The drawing under review shows one solid part. Ordinate dimensions are in mm from its lowest x, y, z. A direction names the side the tool comes from. Round coordinates to 2 decimals unless told otherwise and drop trailing zeros. Write each loop counter-clockwise with the first axis right and the second up, starting at its lowest first coordinate (ties: lowest second). Pieces come first, ordered by that corner, then holes. Notation, with made-up numbers: (62, 20) -> (69, 20) arc R24 cw to (69, 51) -> close; hole circle Ø5 at (21.25, 19.5). An arc over 180 degrees is marked (long way). Use CSV: the item, a comma, the result in double quotes. Start each with the question number.
1) Machinability: for the marked faces 1, 2, 3, 4 and 5, which of the approach directions +Z, -Z, +X, -X, +Y, -Y give a long, thin tool a straight path to every point of the face, cutting with its end or side? Answer none if there is none.
2) Take a section at B-B, the plane y = 62.5. Give the boundary of the cut face in (x, z), then the cut area to 3 significant figures.
3) Take a section at A-A, the plane x = 49. Give the boundary of the cut face in (y, z), then the cut area to 3 significant figures.
4) Take a section at C-C, the plane x = 15. Give the boundary of the cut face in (y, z).
5) Wall thickness on probe 1 along Y at (x, z) = (94.5, 7.5); probe 2 along Z at (x, y) = (33, 61.5); probe 3 along X at (y, z) = (20.5, 2.5): over which ranges is each line inside the solid? List them lowest first. Write a range as [from, to].
6) For pin 1 Ø0.8 at (x, y) = (81.5, 1) entering from +Z; pin 2 Ø3 at (x, z) = (10.5, 12.5) entering from -Y; pin 3 Ø5 at (x, y) = (60.5, 24.5) entering from +Z, all flat-tipped, find the tip position at first contact; note any pin that passes through.
7) Mouldability with a two-part tool opening along Y and no side actions: class the marked faces 6, 7 and 8 as released by +Y, released by -Y, zero draft, split by the parting line, or undercut.
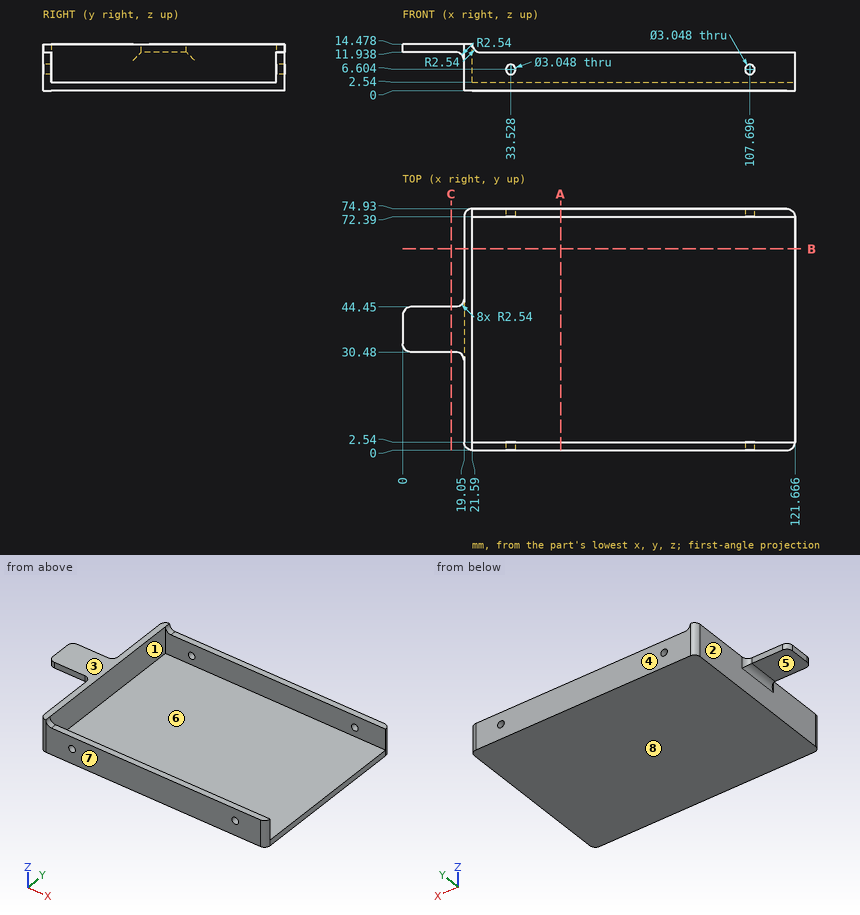
Values found:
1,face 1,"+Z, +X"
1,face 2,"-Z, -X"
1,face 3,"+Z, +X, -X, +Y, -Y"
1,face 4,"+Z, -Z, +X, -X, +Y"
1,face 5,"-Z, -X, +Y, -Y"
2,outline,"(19.05, 0) -> (121.67, 0) -> (121.67, 2.54) -> (21.59, 2.54) -> (21.59, 14.48) -> (19.05, 14.48) -> close"
2,area,"291 mm²"
3,outline,"(0, 0) -> (74.93, 0) -> (74.93, 11.94) -> (72.39, 11.94) -> (72.39, 2.54) -> (2.54, 2.54) -> (2.54, 11.94) -> (0, 11.94) -> close"
3,area,"238 mm²"
4,outline,"(30.48, 11.94) -> (44.45, 11.94) -> (44.45, 14.48) -> (30.48, 14.48) -> close"
5,probe 1,"[0, 2.54], [72.39, 74.93]"
5,probe 2,"[0, 2.54]"
5,probe 3,"[19.05, 121.67]"
6,pin 1,"z = 11.94"
6,pin 2,"y = 30.48"
6,pin 3,"z = 2.54"
7,face 6,"undercut"
7,face 7,"released by -Y"
7,face 8,"zero draft"
